```python
from build123d import *

# Parameters (mm, degrees)
SKETCH1_W           = 50
SKETCH1_H           = 44
SKETCH1_R           = 1.2295
SKETCH1_R_2         = 8.1
BOSS_EXTRUDE1_DEPTH = 5
SKETCH2_W           = 50
SKETCH2_H           = 44
SKETCH2_R           = 18
BOSS_EXTRUDE2_DEPTH = 20
SKETCH4_W           = 70
SKETCH4_H           = 110
BOSS_EXTRUDE3_DEPTH = 3
SKETCH6_W           = 50
SKETCH6_H           = 44
BOSS_EXTRUDE4_DEPTH = 15
FILLET1_R           = 10
FILLET3_R           = 5


with BuildPart() as part:
    # Sketch1 → Boss-Extrude1 (new body)
    with BuildSketch(Plane.XY.offset(45.685001235)):
        with Locations((-11.17428291, 8.97761735)):
            Rectangle(SKETCH1_W, SKETCH1_H)
        with Locations((-11.17428291, 22.97761735)):
            Circle(SKETCH1_R, mode=Mode.SUBTRACT)
        with Locations((2.82571709, 8.97761735)):
            Circle(SKETCH1_R, mode=Mode.SUBTRACT)
        with Locations((-11.17428291, -5.02238265)):
            Circle(SKETCH1_R, mode=Mode.SUBTRACT)
        with Locations((-25.17428291, 8.97761735)):
            Circle(SKETCH1_R, mode=Mode.SUBTRACT)
        with Locations((-11.17428291, 8.97761735)):
            Circle(SKETCH1_R_2, mode=Mode.SUBTRACT)
    extrude(amount=BOSS_EXTRUDE1_DEPTH)

    # Sketch2 → Boss-Extrude2 (add)
    with BuildSketch(Plane(origin=(0, 0, 45.685001235), x_dir=(-1, 0, 0), z_dir=(0, 0, -1))):
        with Locations((11.17428291, 8.97761735)):
            Rectangle(SKETCH2_W, SKETCH2_H)
        with Locations((11.17428291, 8.97761735)):
            Circle(SKETCH2_R, mode=Mode.SUBTRACT)
    extrude(amount=BOSS_EXTRUDE2_DEPTH)

    # Sketch4 → Boss-Extrude3 (add)
    with BuildSketch(Plane.XZ.offset(13.02238265)):
        with Locations((-11.17428291, -4.314998765)):
            Rectangle(SKETCH4_W, SKETCH4_H)
    extrude(amount=BOSS_EXTRUDE3_DEPTH)

    # Sketch6 → Boss-Extrude4 (add)
    with BuildSketch(Plane(origin=(0, 0, -14.314998765), x_dir=(-1, 0, 0), z_dir=(0, 0, -1))):
        with Locations((11.17428291, 8.97761735)):
            Rectangle(SKETCH6_W, SKETCH6_H)
        with BuildLine():
            Line((7.67428291, -9.391922655), (14.67428291, -9.391922655))
            ThreePointArc((14.67428291, -9.391922655), (11.17428291, 27.67761735), (7.67428291, -9.391922655))
        make_face(mode=Mode.SUBTRACT)
    extrude(amount=BOSS_EXTRUDE4_DEPTH)

    # Fillet1
    fillet1_edges = [part.edges().sort_by_distance(p)[0] for p in [
        (13.82571709, 30.97761735, -21.814998765),
        (-36.17428291, 30.97761735, -21.814998765),
        (-36.17428291, 30.97761735, 38.185001235),
        (13.82571709, 30.97761735, 38.185001235),
    ]]
    fillet(fillet1_edges, radius=FILLET1_R)

    # Fillet3
    fillet3_edges = [part.edges().sort_by_distance(p)[0] for p in [
        (23.82571709, -14.52238265, -59.314998765),
        (23.82571709, -14.52238265, 50.685001235),
        (-46.17428291, -14.52238265, 50.685001235),
        (-46.17428291, -14.52238265, -59.314998765),
    ]]
    fillet(fillet3_edges, radius=FILLET3_R)


solid = part.part
```
Could you check a few things on this model? Use its own coordinates, in mm. A direction names the side the tool comes from. Coordinates: 2 decimals unless noted, no trailing zeros. Loops run counter-clockwise (first coordinate to the right, second up) from the corner with the lowest first, then second, coordinate; pieces in that order, holes last.
1) Which directions (+Z, -Z, +X, -X, +Y, -Y) give clear straight access to the entire face, cutting with the end or side of a thin tool? Please do faces 4 (the face through (0.3, -5.4, 25.685)), 5 (the face through (-36.174, 4, -22)), 6 (the face through (-11.95, 27.66, -21.71)).
Reported:
face 4: +X, -X, +Y
face 5: +Z, -Z, -X, +Y
face 6: -Z
2) Imagine slicing it at D-D (y = 4). List the corners of the cut face in (x, z) for me (3 decimals).
Reported:
outline: (-36.174, -29.315) - (-29.2, -29.315) - (-29.2, -14.315) - (-36.174, -14.315) - close; (-36.174, 25.685) - (-28.472, 25.685) - (-28.472, 45.685) - (-17.564, 45.685) - (-17.564, 50.685) - (-36.174, 50.685) - close; (-4.784, 45.685) - (6.124, 45.685) - (6.124, 25.685) - (13.826, 25.685) - (13.826, 50.685) - (-4.784, 50.685) - close; (6.851, -29.315) - (13.826, -29.315) - (13.826, -14.315) - (6.851, -14.315) - close
3) Will these pins go through, and if not, where does the flat tip stop? pin 1 Ø7.5 at (y, z) = (-1.5, -19) entering from -X; pin 2 Ø12 at (y, z) = (2, -25) entering from +X; pin 3 Ø1 at (x, y) = (-6, -5) entering from -Z (3 decimals); pin 4 Ø10 at (x, y) = (-24, -8.5) entering from -Z (3 decimals).
Reported:
pin 1: stops at x = -36.17
pin 2: stops at x = 13.83
pin 3: stops at z = 45.685
pin 4: stops at z = -59.315
4) Imagine slicing it at C-C (x = 0). List the corners of the cut face in (y, z) for me (3 decimals).
Reported:
outline: (-16.022, -59.315) - (-13.022, -59.315) - (-13.022, -29.315) - (-6.017, -29.315) - (-6.017, -14.315) - (-13.022, -14.315) - (-13.022, 25.685) - (-5.134, 25.685) - (-5.134, 45.685) - (23.089, 45.685) - (23.089, 25.685) - (30.978, 25.685) - (30.978, 50.685) - (-16.022, 50.685) - close; (23.972, -29.315) - (30.978, -29.315) - (30.978, -14.315) - (23.972, -14.315) - close
5) Imagine slicing it at A-A (z = -27). List the corners of the cut face in (x, y) for me.
Reported:
outline: (-46.17, -16.02) - (23.83, -16.02) - (23.83, -13.02) - (13.83, -13.02) - (13.83, 20.98) arc R10 ccw to (3.83, 30.98) - (-26.17, 30.98) arc R10 ccw to (-36.17, 20.98) - (-36.17, -13.02) - (-46.17, -13.02) - close; hole (-14.67, -9.39) - (-7.67, -9.39) arc R18.7 ccw (long way) to start
6) Please list where these lines run through material, in increasing order: line 1 along Z through (x, y) = (7.5, 2.5) (3 decimals); line 2 along Y through (x, z) = (-11.5, -25); line 3 along Y through (x, z) = (19, -12).
Reported:
line 1: z = -29.315 to -14.315, 25.685 to 50.685
line 2: y = -16.02 to -9.39, 27.67 to 30.98
line 3: y = -16.02 to -13.02
7) Thinking about a two-plate mould opening in Y: for faces 1 (the face through (-11.3, 24.2, 48.2)), 2 (the face through (23.826, -15, -5)), 3 (the face through (-33.323, 27.971, -21.92)), which applies, released by +Y, released by -Y, zero draft, split by the parting line, or undercut?
Reported:
face 1: undercut
face 2: zero draft
face 3: released by +Y
8) Imagine slicing it at B-B (y = 12.5). List the corners of the cut face in (x, z) for me (3 decimals).
Reported:
outline: (-36.174, -29.315) - (-29.54, -29.315) - (-29.54, -14.315) - (-36.174, -14.315) - close; (-36.174, 25.685) - (-28.826, 25.685) - (-28.826, 45.685) - (-18.468, 45.685) - (-18.468, 50.685) - (-36.174, 50.685) - close; (-3.88, 45.685) - (6.478, 45.685) - (6.478, 25.685) - (13.826, 25.685) - (13.826, 50.685) - (-3.88, 50.685) - close; (7.191, -29.315) - (13.826, -29.315) - (13.826, -14.315) - (7.191, -14.315) - close
